Check sheet for the modelled part. Datum: model origin and axes. Units: mm. Face numbers are marked on the shaded views. A direction names the side the tool comes from. Round coordinates to 2 decimals unless told otherwise and drop trailing zeros. Write each loop counter-clockwise with the first axis right and the second up, starting at its lowest first coordinate (ties: lowest second). Pieces come first, ordered by that corner, then holes.
Item 1: Depth check by flat-ended pin: pin 1 (2 mm diameter, centred on x = 3, y = 8.5, fed in from -Z); pin 2 (2 mm diameter, centred on x = 2, y = 16, fed in from -Z) (3 decimals). Enter the tip coordinate at first touch or a pass-through.
Item 2: Material ranges on line 1 along Y through (x, z) = (0, 6.5); line 2 along Z through (x, y) = (-0.5, 13.25); line 3 along Z through (x, y) = (-1.5, 12), recorded low to high.
Item 3: Section check C-C, the plane x = 4.75. Record the cut outline in (y, z).
Item 4: Section check D-D, the plane y = 2. Record the cut outline in (x, z).
Item 5: Section check B-B, the plane y = 10.5. Record the cut outline in (x, z), plus the area to 3 significant figures.
Item 6: Set-up check for the marked faces 1 and 2: record each of +Z, -Z, +X, -X, +Y, -Y from which the full face is reachable in a straight line by a thin tool's end or side.
Item 7: Section check A-A, the plane z = 0. Record the cut outline in (x, y), plus the area to 3 significant figures.
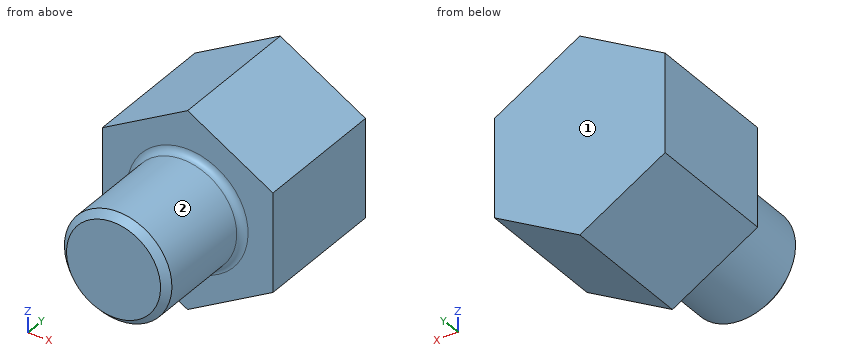
from build123d import *

# Parameters (mm, degrees)
BOSS_EXTRUDE1_DEPTH = 18
SKETCH2_R           = 11.041955005
SKETCH2_R_2         = 4
CUT_EXTRUDE1_DEPTH  = 8
CHAMFER1_SIZE       = 0.5
FILLET1_R           = 0.5


with BuildPart() as part:
    # Sketch1 → Boss-Extrude1 (new body)
    with BuildSketch(Plane(origin=(0, 0, 0), x_dir=(1, 0, 0), z_dir=(0, 1, 0))):
        Polygon((6.35, 3.666174209), (0, 7.332348419), (-6.35, 3.666174209), (-6.35, -3.666174209), (0, -7.332348419), (6.35, -3.666174209), align=None)
    extrude(amount=BOSS_EXTRUDE1_DEPTH)

    # Sketch2 → Cut-Extrude1 (cut)
    with BuildSketch(Plane.XZ):
        Circle(SKETCH2_R)
        with Locations(Location((0, 0, 0), (0, 0, 270))):
            Circle(SKETCH2_R_2, mode=Mode.SUBTRACT)
    extrude(amount=-CUT_EXTRUDE1_DEPTH, mode=Mode.SUBTRACT)

    # Chamfer1
    chamfer1_edges = [part.edges().sort_by_distance(p)[0] for p in [
        (0, 0, 4),
    ]]
    chamfer(chamfer1_edges, length=CHAMFER1_SIZE)

    # Fillet1
    fillet1_edges = [part.edges().sort_by_distance(p)[0] for p in [
        (0, 8, 4),
    ]]
    fillet(fillet1_edges, radius=FILLET1_R)


solid = part.part
Values found:
1. pin 1: stops at z = -6.18
1. pin 2: stops at z = -6.755
2. line 1: y = 8 to 18
2. line 2: z = -7.04 to 7.04
2. line 3: z = -6.47 to 6.47
3. outline: (8, -4.59) - (18, -4.59) - (18, 4.59) - (8, 4.59) - close
4. outline: circle Ø8 at (0, 0)
5. outline: (-6.35, -3.67) - (0, -7.33) - (6.35, -3.67) - (6.35, 3.67) - (0, 7.33) - (-6.35, 3.67) - close
5. area: 140 mm2
6. face 1: +Z, -Z, +X, -X, +Y
6. face 2: -Y
7. outline: (-6.35, 8) - (-4.5, 8) arc R0.5 cw to (-4, 7.5) - (-4, 0.5) - (-3.5, 0) - (3.5, 0) - (4, 0.5) - (4, 7.5) arc R0.5 cw to (4.5, 8) - (6.35, 8) - (6.35, 18) - (-6.35, 18) - close
7. area: 191 mm2
